Work out the finished part from the listing and answer in its coordinate system (mm). A direction names the side the tool comes from. Round coordinates to 2 decimals unless told otherwise and drop trailing zeros. Loops run counter-clockwise (first coordinate to the right, second up) from the corner with the lowest first, then second, coordinate; pieces in that order, holes last. Notation, with made-up numbers: M 78,-27.5 L 123,-27.5 A23 ccw 123,-7.5 Z; hole C -30,-32 d1. An arc over 180 degrees is marked long. One line per item, written item: value.
```python
from build123d import *

# Parameters (mm, degrees)
F1_DEPTH    = 5.6
F0_R        = 2.25
F0_W        = 8
F0_H        = 10.336498642
F2_DEPTH    = 3
F3_T1_DEPTH = 20.6876119668
F3_T3_DEPTH = 21.0057116197
F3_T6_ANGLE = 66.24239892
F3_T8_ANGLE = 176.3763770041


# Not quite as in the source:
# - a fillet or chamfer that OpenCascade refuses, or shapes differently, is made with other operations: its cross-section is extruded or revolved along the edge and cut away or added


with BuildPart() as f1:
    # F0 (on Front) → F1 (new body)
    with BuildSketch(Plane.XZ):
        with BuildLine():
            Line((-10.5, 5.086498642), (-12.5051002221, 5.086498642))
            ThreePointArc((-12.5051002221, 5.086498642), (-13.4997099623, -0.0884925705), (-12.4373429638, -5.25))
            Line((-12.4373429638, -5.25), (-10.5, -5.25))
            Line((-10.5, -5.25), (-10.5, 5.086498642))
        make_face()
    extrude(amount=F1_DEPTH)



with BuildPart() as f1b:
    # F0 (on Front) → F1, piece 2 (new body)
    with BuildSketch(Plane.XZ):
        with BuildLine():
            Line((3.5006113976, 5.086498642), (-2.5, 5.086498642))
            Line((-2.5, 5.086498642), (-2.5, -5.25))
            Line((-2.5, -5.25), (3.2502690029, -5.25))
            ThreePointArc((3.2502690029, -5.25), (6.1728759577, -0.1495025156), (3.5006113976, 5.086498642))
        make_face()
        Circle(F0_R, mode=Mode.SUBTRACT)
    extrude(amount=F1_DEPTH)


with BuildPart() as f1_1:
    add(f1.part)

    add(f1b.part)  # F2 merges F1b
    # F0 (on Front) → F2 (join)
    with BuildSketch(Plane.XZ):
        with BuildLine():
            Line((-10.5, 5.086498642), (-12.5051002221, 5.086498642))
            ThreePointArc((-12.5051002221, 5.086498642), (-13.4997099623, -0.0884925705), (-12.4373429638, -5.25))
            Line((-12.4373429638, -5.25), (-10.5, -5.25))
            Line((-10.5, -5.25), (-10.5, 5.086498642))
        make_face()
        with Locations((-6.5, -0.081750679)):
            Rectangle(F0_W, F0_H)
        with BuildLine():
            Line((3.5006113976, 5.086498642), (-2.5, 5.086498642))
            Line((-2.5, 5.086498642), (-2.5, -5.25))
            Line((-2.5, -5.25), (3.2502690029, -5.25))
            ThreePointArc((3.2502690029, -5.25), (6.1728759577, -0.1495025156), (3.5006113976, 5.086498642))
        make_face()
        Circle(F0_R, mode=Mode.SUBTRACT)
    extrude(amount=-F2_DEPTH)

    # F3: fillet of radius 1 on 4 edges, made by hand

    # F3_s2 → F3_t1 (cut)
    with BuildSketch(Plane.YZ.offset(-14.9373429638)):
        with BuildLine():
            ThreePointArc((3, -4.25), (2.7071067812, -4.9571067812), (2, -5.25))
            Line((2, -5.25), (3, -5.25))
            Line((3, -5.25), (3, -4.25))
        make_face()
    extrude(amount=F3_T1_DEPTH, mode=Mode.SUBTRACT)

    # F3_s4 → F3_t3 (cut)
    with BuildSketch(Plane.YZ.offset(-15.0051002221)):
        with BuildLine():
            ThreePointArc((3, 4.086498642), (2.7071067812, 4.7936054231), (2, 5.086498642))
            Line((2, 5.086498642), (3, 5.086498642))
            Line((3, 5.086498642), (3, 4.086498642))
        make_face()
    extrude(amount=F3_T3_DEPTH, mode=Mode.SUBTRACT)

    # F3_s5 → F3_t6 (revolve, cut)
    with BuildSketch(Plane(origin=(0, 0, 0), x_dir=(0, 1, 0), z_dir=(0.5409102149, 0, 0.8410803406))):
        with BuildLine():
            ThreePointArc((3, 12.5), (2.7071067812, 13.2071067812), (2, 13.5))
            Line((2, 13.5), (3, 13.5))
            Line((3, 13.5), (3, 12.5))
        make_face()
    revolve(axis=Axis((0, 3, 0), (0, -1, 0)), revolution_arc=F3_T6_ANGLE, mode=Mode.SUBTRACT)

    # F3_s7 → F3_t8 (revolve, cut)
    with BuildSketch(Plane(origin=(0, 0, 0), x_dir=(0, 1, 0), z_dir=(-0.9888894164, 0, -0.148653026))):
        with BuildLine():
            ThreePointArc((2, 6.1746861128), (2.7071067812, 5.881792894), (3, 5.1746861128))
            Line((3, 5.1746861128), (3, 6.1746861128))
            Line((3, 6.1746861128), (2, 6.1746861128))
        make_face()
    revolve(axis=Axis((0, 3, 0), (0, -1, 0)), revolution_arc=F3_T8_ANGLE, mode=Mode.SUBTRACT)


solid = f1_1.part
```
1) Find section C-C (x = 0). Give the vertices of the cut face in (y, z).
Check values:
outline: M -5.6,-5.25 L 2,-5.25 A1 ccw 3,-4.25 L 3,-2.25 L -5.6,-2.25 Z; M -5.6,2.25 L 3,2.25 L 3,4.09 A1 ccw 2,5.09 L -5.6,5.09 Z
2) Find section A-A (y = -3). Give the vertices of the cut face in (x, z).
Check values:
outline: M -12.51,5.09 A13.5 ccw -12.44,-5.25 L -10.5,-5.25 L -10.5,5.09 Z; M -2.5,-5.25 L 3.25,-5.25 A6.17 ccw 3.5,5.09 L -2.5,5.09 Z; hole C 0,0 d4.5
3) Find the intervals of material crossed by probe 1 along Z at (x, y) = (0, -1.75); probe 2 along X at (y, z) = (-0.5, 0.75); probe 3 along Y at (x, z) = (-3, -2), in increasing order. Write a range as from..to.
Check values:
probe 1: -5.25..-2.25, 2.25..5.09
probe 2: -13.48..-10.5, -2.5..-2.12, 2.12..6.13
probe 3: 0..3
4) Find section D-D (y = 1.5). Give the vertices of the cut face in (x, z), then the cut area to 3 significant figures.
Check values:
outline: M -12.51,5.09 A13.5 ccw -12.44,-5.25 L 3.25,-5.25 A6.17 ccw 3.5,5.09 Z; hole C 0,0 d4.5
area: 175 mm2
5) Each of these flat-tipped pins is pushed along its axis until it touches: pin 1 (5 mm diameter, centred on x = -5.5, z = 1, fed in from -Y); pin 2 (1.5 mm diameter, centred on y = 1.5, z = -1, fed in from -X); pin 3 (3 mm diameter, centred on y = -3, z = 2, fed in from +X). Where does it stop, or does it pass through?
Check values:
pin 1: y = 0
pin 2: x = -13.5
pin 3: x = 6.15
6) The mould has two halves that part along X. Classify faces 1 (the face through (-13.5, -1.9, 0)), 2 (the face through (-0.29, -1.24, 2.23)), 3 (the face through (-3, 1, -5.25)): +X half, -X half, draft (parallel to the pull), parting line (faces both ways), or undercut.
Check values:
face 1: -X half
face 2: undercut
face 3: draft
7) Find section B-B (z = 0). Give the vertices of the cut face in (x, y).
Check values:
outline: M -13.5,-5.6 L -10.5,-5.6 L -10.5,0 L -2.5,0 L -2.5,-5.6 L -2.25,-5.6 L -2.25,3 L -12.5,3 A1 ccw -13.5,2 Z; M 2.25,-5.6 L 6.17,-5.6 L 6.17,2 A1 ccw 5.17,3 L 2.25,3 Z
8) For faces 4 (the face through (-2.5, -3, 0)), 5 (the face through (-3, 1, 5.086)), determine the directions among +Z, -Z, +X, -X, +Y, -Y from which every point of the face is accessible in a straight line to the end or side of a thin tool.
Check values:
face 4: +Z, -Z, -Y
face 5: +Z, +X, -X, +Y, -Y
